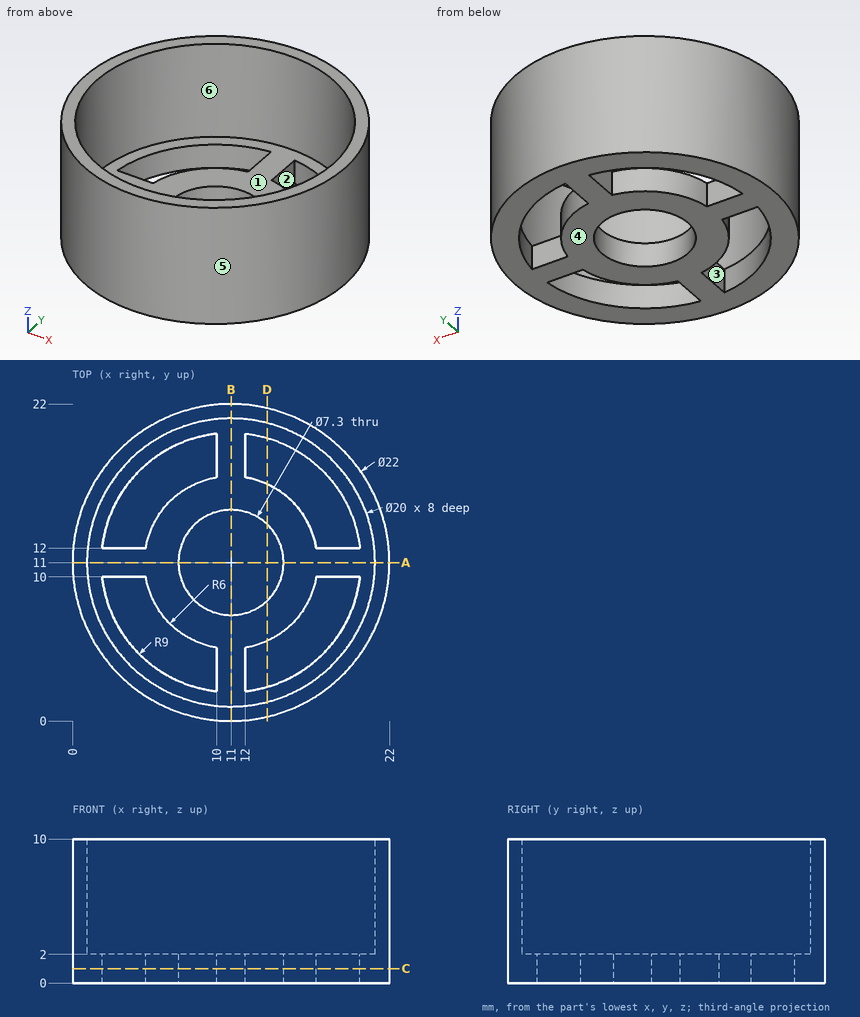
Verification items for this drawing (mm, ordinates from the low corner). A direction names the side the tool comes from. Give positions to 0.01 mm unless a question says otherwise; leave off trailing zeros. Loops run counter-clockwise (first coordinate to the right, second up) from the corner with the lowest first, then second, coordinate; pieces in that order, holes last.
(1) Release check for a two-part mould opening along X. For the marked faces 3, 4, 5 and 6 record: released by +X, released by -X, zero draft, split by the parting line, or undercut.
From the geometry:
face 3: undercut
face 4: zero draft
face 5: split by the parting line
face 6: undercut
(2) Set-up check for the marked faces 1 and 2: record each of +Z, -Z, +X, -X, +Y, -Y from which the full face is reachable in a straight line by a thin tool's end or side.
From the geometry:
face 1: +Z
face 2: +Z, -Z
(3) Section check C-C on z = 1. Record the cut outline in (x, y).
From the geometry:
outline: circle Ø22 at (11, 11); hole (2.06, 10) arc R9 ccw to (10, 2.06) - (10, 5.08) arc R6 cw to (5.08, 10) - close; hole (2.06, 12) - (5.08, 12) arc R6 cw to (10, 16.92) - (10, 19.94) arc R9 ccw to start; hole circle Ø7.3 at (11, 11); hole (12, 2.06) arc R9 ccw to (19.94, 10) - (16.92, 10) arc R6 cw to (12, 5.08) - close; hole (12, 16.92) arc R6 cw to (16.92, 12) - (19.94, 12) arc R9 ccw to (12, 19.94) - close
(4) Thickness scan on L1, parallel to Y at x = 11, z = 0.8; L2, parallel to Y at x = 11, z = 4.5; L3, parallel to Y at x = 3, z = 1. Record the ranges inside material, lowest first.
From the geometry:
L1: y = 0 to 7.35, 14.65 to 22
L2: y = 0 to 1, 21 to 22
L3: y = 3.45 to 6.88, 10 to 12, 15.12 to 18.55
(5) Section check D-D on x = 13.5. Record the cut outline in (y, z).
From the geometry:
outline: (0.29, 0) - (2.35, 0) - (2.35, 2) - (1.32, 2) - (1.32, 10) - (0.29, 10) - close; (5.55, 0) - (8.34, 0) - (8.34, 2) - (5.55, 2) - close; (13.66, 0) - (16.45, 0) - (16.45, 2) - (13.66, 2) - close; (19.65, 0) - (21.71, 0) - (21.71, 10) - (20.68, 10) - (20.68, 2) - (19.65, 2) - close
(6) Section check A-A on y = 11. Record the cut outline in (x, z), then the cut area to 3 significant figures.
From the geometry:
outline: (0, 0) - (7.35, 0) - (7.35, 2) - (1, 2) - (1, 10) - (0, 10) - close; (14.65, 0) - (22, 0) - (22, 10) - (21, 10) - (21, 2) - (14.65, 2) - close
area: 45.4 mm2
(7) Depth check by flat-ended pin: pin 1 Ø0.6 at (y, z) = (3.5, 0.5) entering from +X; pin 2 Ø1 at (y, z) = (3.5, 1) entering from -X; pin 3 Ø2 at (y, z) = (18.5, 1) entering from +X. Enter the tip coordinate at first touch or a pass-through.
From the geometry:
pin 1: stops at x = 19.32
pin 2: stops at x = 2.51
pin 3: stops at x = 19.87
